Can you work these out from the model? Positions are in its coordinate system, mm. A direction names the side the tool comes from. Coordinates: 2 decimals unless noted, no trailing zeros. Loops run counter-clockwise (first coordinate to the right, second up) from the corner with the lowest first, then second, coordinate; pieces in that order, holes last. Notation, with made-up numbers: (77, 74) -> (89, 74) arc R22 ccw to (89, 94) -> close; hole circle Ø8 at (86.25, -24). An arc over 180 degrees is marked (long way). Use one line per item in the form item = value. Start each with the question number.
(1) Imagine slicing it at B-B (z = -1). List the corners of the cut face in (x, y) for me, plus the area to 3 significant figures.
(2) On a 3-axis mill with a long thin cutter (end or side, diameter ignored), from which of +Z, -Z, +X, -X, +Y, -Y can I reach the whole of each face in a straight line? I mean faces 4 (the flat face through (-4, 4, 0)), 5 (the flat face through (0, 0, -2)). Say none if no direction works.
(3) I need wall thicknesses on line 1 (Y direction, x = 0, z = 4.45); line 2 (Z direction, x = 0.5, y = 0.75); line 3 (Z direction, x = -7.75, y = 4). Which ranges of each line are inside material? Lowest first, please. Write a range as [from, to].
(4) Thinking about a two-plate mould opening in X: for faces 1 (the flat face through (2.2, -2.2, 0.4)), 2 (the cylindrical face through (-1.825, -1.4, 1.881)), 3 (the cylindrical face through (-1.08, -4.88, 0.2)), which applies, released by +X, released by -X, zero draft, split by the parting line, or undercut?
(5) Imagine slicing it at A-A (z = 4.75). List the corners of the cut face in (x, y) for me, plus the area to 3 significant figures.
(6) I'm going to push flat-ended pins straight in: pin 1 (3 mm diameter, centred on x = 0, y = 0, fed in from +Z); pin 2 (5 mm diameter, centred on x = 3.5, y = 11.5, fed in from +Z); pin 3 (9 mm diameter, centred on x = -6.5, y = -5.5, fed in from +Z); pin 4 (1 mm diameter, centred on x = 4, z = 3.5, fed in from +Y). Where does each tip first touch, or does it pass through?
```python
from build123d import *

# Parameters (mm, degrees)
F0_R     = 2.9
F1_DEPTH = 7
F2_T     = -0.6
F0_R_2   = 15
F0_R_3   = 5
F3_DEPTH = 2
F4_R     = 1.99999
F7_R     = 0.3
F8_DEPTH = 0.4


# Not quite as in the source:
# - a fillet or chamfer is up to 0.001 mm smaller than in the source, because OpenCascade refuses the exact size


with BuildPart() as f1:
    # F0 (on Top) → F1 (new body)
    with BuildSketch(Plane.XY):
        Circle(F0_R)
    extrude(amount=F1_DEPTH)

    # F2
    f2_openings = [f1.faces().sort_by_distance(p)[0] for p in [
        (0, 0, 7),
    ]]
    offset(amount=F2_T, openings=f2_openings)

    # F0 (on Top) → F3 (join)
    with BuildSketch(Plane.XY):
        Circle(F0_R_2)
        Circle(F0_R_3, mode=Mode.SUBTRACT)
        Circle(F0_R_3)
        Circle(F0_R, mode=Mode.SUBTRACT)
        Circle(F0_R)
    extrude(amount=-F3_DEPTH)

    # F4 (radius 2 in the source; OpenCascade refuses exactly that, so slightly less here)
    f4_edges = [f1.edges().sort_by_distance(p)[0] for p in [
        (-15, 0, -2),
    ]]
    fillet(f4_edges, radius=F4_R)

    # F5 (on Front) → F6 (revolve, cut)
    with BuildSketch(Plane.XZ):
        with BuildLine():
            ThreePointArc((2.175, 3.5), (2.2116116524, 3.4116116524), (2.3, 3.375))
            Line((2.3, 3.375), (2.3, 3.5))
            Line((2.3, 3.5), (2.175, 3.5))
        make_face()
        with BuildLine():
            Line((2.3, 3.5), (2.3, 3.375))
            ThreePointArc((2.3, 3.375), (2.3883883476, 3.4116116524), (2.425, 3.5))
            ThreePointArc((2.425, 3.5), (2.3, 3.625), (2.175, 3.5))
            Line((2.175, 3.5), (2.3, 3.5))
        make_face()
    revolve(axis=Axis((0, 0, 1.75), (0, 0, 1)), mode=Mode.SUBTRACT)

    # F7
    f7_edges = [f1.edges().sort_by_distance(p)[0] for p in [
        (-2.3, 0, 3.375),
    ]]
    fillet(f7_edges, radius=F7_R)

    # F0 (on Top) → F8 (join)
    with BuildSketch(Plane.XY):
        Circle(F0_R_3)
        Circle(F0_R, mode=Mode.SUBTRACT)
    extrude(amount=F8_DEPTH)


solid = f1.part
```
Worked out:
q1.outline = circle Ø29.46 at (0, 0)
q1.area = 682 mm2
q2.face_4 = +Z
q2.face_5 = -Z, +X, -X, +Y, -Y
q3.line_1 = [-2.9, -2.3], [2.3, 2.9]
q3.line_2 = [-2, 0.6]
q3.line_3 = [-2, 0]
q4.face_1 = zero draft
q4.face_2 = undercut
q4.face_3 = split by the parting line
q5.outline = circle Ø5.8 at (0, 0); hole circle Ø4.6 at (0, 0)
q5.area = 9.80 mm2
q6.pin_1 = 0.6
q6.pin_2 = 0
q6.pin_3 = 0.4
q6.pin_4 = through
